Autodesk Inventor part; units mm, degrees
ref_plane "YZ Plane" through (0, 0, 0) normal (1, 0, 0) x (0, 1, 0)
ref_plane "XZ Plane" through (0, 0, 0) normal (0, 1, 0) x (-1, 0, 0)
ref_plane "XY Plane" through (0, 0, 0) normal (0, 0, 1) x (1, 0, 0)
sketch "Sketch1" plane through (0, 0, 0) normal (1, 0, 0) x (0, 1, 0)
  line L0 (0, 0) -> (14.5, 0)
  line L1 (14.5, 0) -> (14.5, -14.5)
  line L2 (14.5, -14.5) -> (0, -14.5)
  line L3 (0, -14.5) -> (0, 0)
  dimension "d5" = 14.5
  dimension "d6" = 14.5
extrude "Extrusion1" add sketch "Sketch1" along normal blind 6.88
fillet "Fillet1" radius 1 10 edges at (0, 0, -7.25) (0, 7.25, -14.5) (3.44, 0, -14.5) (6.88, 7.25, -14.5) (6.88, 0, -7.25) (6.88, 7.25, 0) (0, 7.25, 0) (3.44, 0, 0) (0, 14.5, -7.25) (6.88, 14.5, -7.25)
properties part number "battery_1S_100mAh_no_prot"
The model under review builds one solid part; all positions refer to its coordinate system, in mm. Give positions to 0.01 mm unless a question says otherwise; leave off trailing zeros. Order: outer loops, then holes, each group sorted by start corner. A loop starts at its lowest first (then second) coordinate and runs counter-clockwise, first axis right, second up. Notation, with made-up numbers: (-39, 46.25) - (-17, 46.25) arc R19 ccw to (-17, 71.25) - close; hole circle Ø10 at (43, 57.5). An arc over 180 degrees is marked (long way). Use CSV: the item, a comma, the result in double quotes. Start each with the question number.
Q1. We need section A-A, the plane x = 6.5. Write out the cut boundary in (y, z), and give its area (3 significant figures).
Q2. Clearance check with a flat-ended pin moving along its axis: pin 1 Ø3 at (x, z) = (5.5, -5) entering from -Y. State where the tip first meets the part, or that it passes through.
Q3. To check wall thickness, follow line 1 along Z through (x, y) = (6, 13); line 2 along Y through (x, z) = (6, -1); line 3 along Z through (x, y) = (0.5, 6.5). State the ranges of each line that lie inside material, in increasing order. Write a range as [from, to].
Outcome:
1,outline,"(0.22, -13.5) arc R0.78 ccw to (1, -14.28) - (14.28, -14.28) - (14.28, -0.22) - (1, -0.22) arc R0.78 ccw to (0.22, -1) - close"
1,area,"198 mm^2"
2,pin 1,"stops at y = 0"
3,line 1,"z = [-14.49, -0.01]"
3,line 2,"y = [0.01, 14.49]"
3,line 3,"z = [-14.37, -0.13]"
